Autodesk Inventor part; units mm, degrees
ref_plane "YZ Plane" through (0, 0, 0) normal (1, 0, 0) x (0, 1, 0)
ref_plane "XZ Plane" through (0, 0, 0) normal (0, 1, 0) x (-1, 0, 0)
ref_plane "XY Plane" through (0, 0, 0) normal (0, 0, 1) x (1, 0, 0)
sketch "Sketch1" plane through (0, 0, 0) normal (0, 0, 1) x (1, 0, 0)
  arc A0 (0, 9.2) -> (0, -9.2) centre (0, 0) ccw
  arc A1 (18.6, -9.2) -> (18.6, 9.2) centre (18.6, 0) ccw
  line L0 (0, 9.2) -> (18.6, 9.2)
  line L1 (0, -9.2) -> (18.6, -9.2)
  dimension "d0" = 18.4
  dimension "d1" = 18.4
  dimension "d2" = 18.6
extrude "Extrusion1" add sketch "Sketch1" along normal blind 65
sketch "Sketch2" plane through (0, 0, 65) normal (0, 0, 1) x (1, 0, 0)
  line L0 (18.6, 9.2) -> (0, 9.2)
  arc A0 (0, 9.2) -> (0, -9.2) centre (0, 0) ccw
  line L1 (0, -9.2) -> (18.6, -9.2)
  arc A1 (18.6, -9.2) -> (18.6, 9.2) centre (18.6, 0) ccw
  line L2 (0, 5.2) -> (18.6, 5.2)
  arc A2 (18.6, -5.2) -> (18.6, 5.2) centre (18.6, 0) ccw
  line L3 (18.6, -5.2) -> (0, -5.2)
  arc A3 (0, 5.2) -> (0, -5.2) centre (0, 0) ccw
  dimension "d7" = 4
extrude "Extrusion2" add sketch "Sketch2" along normal blind 0.1
sketch "Sketch3" plane through (0, 0, 0) normal (0, 0, -1) x (-1, 0, 0)
  line L0 (-18.6, 9.2) -> (0, 9.2)
  arc A0 (-18.6, 9.2) -> (-18.6, -9.2) centre (-18.6, 0) ccw
  line L1 (0, -9.2) -> (-18.6, -9.2)
  arc A1 (0, -9.2) -> (0, 9.2) centre (0, 0) ccw
  line L2 (0, 5.2) -> (-18.6, 5.2)
  arc A2 (-18.6, 5.2) -> (-18.6, -5.2) centre (-18.6, 0) ccw
  line L3 (-18.6, -5.2) -> (0, -5.2)
  arc A3 (0, -5.2) -> (0, 5.2) centre (0, 0) ccw
  dimension "d8" = 4
extrude "Extrusion3" add sketch "Sketch3" along normal blind 0.1
sketch "Sketch4" plane through (0, 9.2, 65.1) normal (0, 1, 0) x (1, 0, 0)
  point P0 (0, 65.1)
sketch "Sketch5" plane through (0, 9.2, 65.1) normal (0, 1, 0) x (1, 0, 0)
  line L0 (25.672, 60.4824) -> (25.672, 5.7019) construction
  line L1 (25.672, 5.7019) -> (-6.5778, 5.7019) construction
  line L2 (-6.5778, 5.7019) -> (-6.5778, 60.4824) construction
  line L3 (-6.5778, 60.4824) -> (25.672, 60.4824) construction
  point P0 (0, 65.1)
decal "Decal1"
sketch "Sketch6" plane through (0, 0, 65.1) normal (0, 0, 1) x (1, 0, 0)
  arc A0 (18.6, -5.2) -> (18.6, 5.2) centre (18.6, 0) ccw
  line L0 (18.6, -5.2) -> (0, -5.2)
  arc A1 (0, 5.2) -> (0, -5.2) centre (0, 0) ccw
  line L1 (0, 5.2) -> (18.6, 5.2)
  line L2 (18.6, 9.2) -> (0, 9.2)
  arc A2 (0, 9.2) -> (0, -9.2) centre (0, 0) ccw
  line L3 (0, -9.2) -> (18.6, -9.2)
  arc A3 (18.6, -9.2) -> (18.6, 9.2) centre (18.6, 0) ccw
properties part number "Battery Pack"
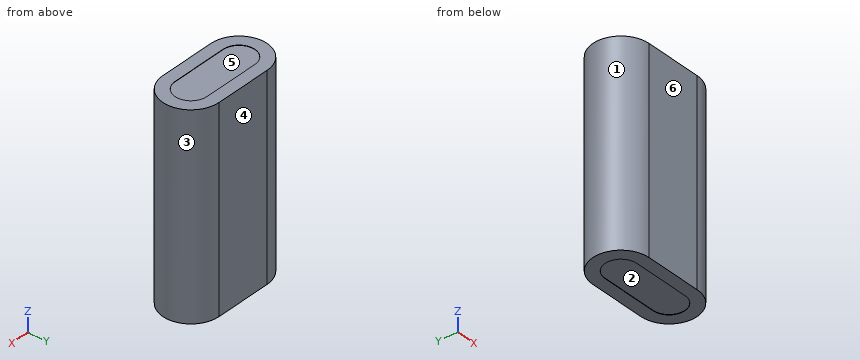
Geometry check sheet. Reference: the model listing, model coordinates, mm. Face numbers are marked on the shaded views. A direction names the side the tool comes from. Give positions to 0.01 mm unless a question says otherwise; leave off trailing zeros. Write each loop counter-clockwise with the first axis right and the second up, starting at its lowest first coordinate (ties: lowest second). Pieces come first, ordered by that corner, then holes.
1) Section check A-A, the plane y = -3.25. Record the boundary of the cut face in (x, z), and give its area (3 significant figures).
2) Access from +Z, -Z, +X, -X, +Y, -Y to the whole of each face (thin tool, end or side, straight path). Record for the marked faces 5 and 6.
3) Section check C-C, the plane x = -7. Record the boundary of the cut face in (y, z), and give its area (3 significant figures).
4) Section check B-B, the plane z = 56. Record the boundary of the cut face in (x, y).
5) Material ranges on L1, parallel to X at y = 0.5, z = 34; L2, parallel to Z at x = 14, y = 0.25; L3, parallel to Y at x = 19, z = 10, recorded low to high.
6) Release check for a two-part mould opening along X. For the marked faces 1, 2, 3 and 4 record: pulls with the +X half, pulls with the -X half, needs draft (parallel to the pull), parting line crosses it, or undercut.
7) Gauge pin test, flat ends, axial feed: pin 1 (8.5 mm diameter, centred on x = 8.5, y = 1.5, fed in from +Z); pin 2 (3 mm diameter, centred on y = -5, z = 38, fed in from -X); pin 3 (3 mm diameter, centred on x = 8, y = -1.5, fed in from -Z); pin 4 (2 mm diameter, centred on x = 2, y = 2.5, fed in from +Z). Record the tip position at first contact, or that the pin passes through.
Computed:
1. outline: (-8.61, -0.1) - (-4.06, -0.1) - (-4.06, 0) - (22.66, 0) - (22.66, -0.1) - (27.21, -0.1) - (27.21, 65.1) - (22.66, 65.1) - (22.66, 65) - (-4.06, 65) - (-4.06, 65.1) - (-8.61, 65.1) - close
1. area: 2,330 mm2
2. face 5: +Z
2. face 6: +Z, -Z, +X, -X, -Y
3. outline: (-5.97, -0.1) - (5.97, -0.1) - (5.97, 65.1) - (-5.97, 65.1) - close
3. area: 778 mm2
4. outline: (0, -9.2) - (18.6, -9.2) arc R9.2 ccw to (18.6, 9.2) - (0, 9.2) arc R9.2 ccw to start
5. L1: x = -9.19 to 27.79
5. L2: z = 0 to 65
5. L3: y = -9.19 to 9.19
6. face 1: pulls with the -X half
6. face 2: undercut
6. face 3: pulls with the +X half
6. face 4: needs draft
7. pin 1: stops at z = 65.1
7. pin 2: stops at x = -8.51
7. pin 3: stops at z = 0
7. pin 4: stops at z = 65
